For this review, use the dimensioned drawing (mm, ordinates from the lowest corner) and the shaded views. Round coordinates to 2 decimals unless told otherwise and drop trailing zeros. Order: outer loops, then holes, each group sorted by start corner. A loop starts at its lowest first (then second) coordinate and runs counter-clockwise, first axis right, second up. Notation, with made-up numbers: (81, 89.25) -> (91, 89.25) arc R19 cw to (91, 114.25) -> close; hole circle Ø10 at (-22, 10). An arc over 180 degrees is marked (long way). Answer in a Markdown table with one row per item.
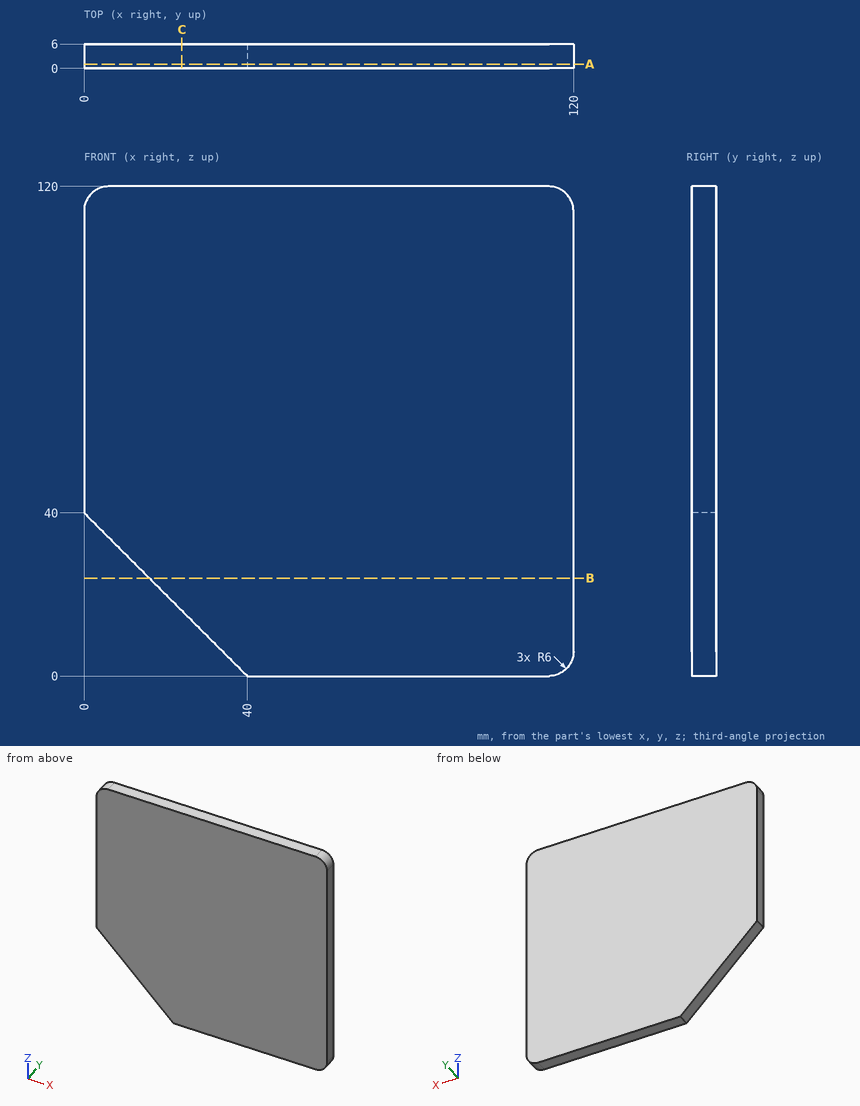
Q1. Take a section at A-A, the plane y = 1.05. Write out the cut boundary in (x, z).
Answer key:
| item | result |
|---|---|
| outline | (0, 40) -> (40, 0) -> (114, 0) arc R6 ccw to (120, 6) -> (120, 114) arc R6 ccw to (114, 120) -> (6, 120) arc R6 ccw to (0, 114) -> close |
Q2. Clearance check with a flat-ended pin moving along its axis: pin 1 Ø2 at (x, z) = (24, 73.5) entering from -Y. State where the tip first meets the part, or that it passes through.
Answer key:
| item | result |
|---|---|
| pin 1 | stops at y = 0 |
Q3. Take a section at C-C, the plane x = 24. Write out the cut boundary in (y, z), then the cut area to 3 significant figures.
Answer key:
| item | result |
|---|---|
| outline | (0, 16) -> (6, 16) -> (6, 120) -> (0, 120) -> close |
| area | 624 mm^2 |
Q4. Take a section at B-B, the plane z = 24. Write out the cut boundary in (x, y), then the cut area to 3 significant figures.
Answer key:
| item | result |
|---|---|
| outline | (16, 0) -> (120, 0) -> (120, 6) -> (16, 6) -> close |
| area | 624 mm^2 |
Q5. To check wall thickness, follow probe 1 along Z at (x, y) = (8, 5.4); probe 2 along Z at (x, y) = (8.5, 3.25); probe 3 along X at (y, z) = (0.35, 28). State the ranges of each line that lie inside material, in increasing order.
Answer key:
| item | result |
|---|---|
| probe 1 | z = 32 to 120 |
| probe 2 | z = 31.5 to 120 |
| probe 3 | x = 12 to 120 |
